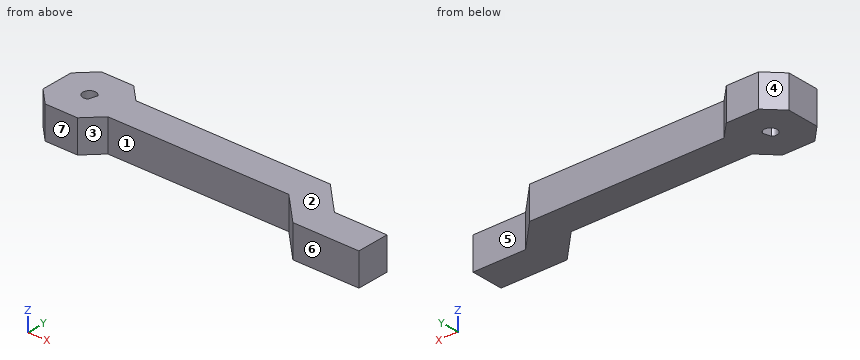
from build123d import *

# Parameters (mm, degrees)
BOSS_EXTRUDE1_DEPTH = 20


with BuildPart() as part:
    # Sketch1 → Boss-Extrude1 (new body)
    with BuildSketch(Plane.XY):
        Polygon((-125.92552771, 40.003004944), (-115.92552771, 50.003004944), (-95.92552771, 50.003004944), (-85.92552771, 40.003003647), (34.07447229, 40.003003647), (52.904699458, 21.17277648), (85.359896376, 21.17277648), (85.359896376, 1.17277648), (44.62042821, 1.17277648), (25.790201043, 20.003003647), (-85.92552771, 20.003003647), (-95.92552771, 10.003004944), (-115.92552771, 10.003004944), (-125.92552771, 20.003004944), align=None)
        with BuildLine():
            Line((-103.718736643, 26.666828512), (-102.339668887, 31.775465524))
            ThreePointArc((-102.339668887, 31.775465524), (-109.787294302, 31.04548218), (-103.718736643, 26.666828512))
        make_face(mode=Mode.SUBTRACT)
    extrude(amount=BOSS_EXTRUDE1_DEPTH)


solid = part.part
Could you check a few things on this model? Use its own coordinates, in mm. Face numbers are marked on the shaded views. A direction names the side the tool comes from. Give positions to 0.01 mm unless a question says otherwise; leave off trailing zeros. Order: outer loops, then holes, each group sorted by start corner. A loop starts at its lowest first (then second) coordinate and runs counter-clockwise, first axis right, second up. Notation, with made-up numbers: (74, 85) -> (101, 85) arc R16 cw to (101, 92) -> close; hole circle Ø6 at (-20, 74). An arc over 180 degrees is marked (long way). Answer in a Markdown table with one row per item. Add a question column.
Item 1: Imagine slicing it at B-B (z = 4.25). List the corners of the cut face in (x, y) for me.
Item 2: For the marked faces 5, 6 and 7, which set-ups out of +Z, -Z, +X, -X, +Y, -Y let a thin tool reach every point of the face, with its end or its side?
Item 3: I'm going to push flat-ended pins straight in: P1, Ø6, axis at x = -4.5, z = 8.5, coming from the +Y side; P2, Ø6, axis at x = 69, z = 10, coming from the +Y side; P3, Ø1, axis at y = 44, z = 12, coming from the +X side; P4, Ø5, axis at x = -105.93, y = 30, coming from the -Z side. Where does each tip first touch, or does it pass through?
Item 4: We'd pull the mould along X, two halves only. Please class the marked faces 1, 2, 3 and 4: pulls with the +X half, pulls with the -X half, needs draft (parallel to the pull), parting line crosses it, or undercut.
Item 5: Imagine slicing it at D-D (y = 6). List the corners of the cut face in (x, z) for me.
Item 6: Imagine slicing it at A-A (y = 16). List the corners of the cut face in (x, z) for me.
Item 7: Imagine slicing it at C-C (x = -100). List the corners of the cut face in (y, z) for me, and give its area (3 significant figures).
Item 8: Please list where these lines run through material, in increasing order: probe 1 along Y at (x, z) = (71, 15.75); probe 2 along Y at (x, z) = (22.5, 17.5); probe 3 along X at (y, z) = (13, 15.5).
Result:
| question | item | result |
|---|---|---|
| 1 | outline | (-125.93, 20) -> (-115.93, 10) -> (-95.93, 10) -> (-85.93, 20) -> (25.79, 20) -> (44.62, 1.17) -> (85.36, 1.17) -> (85.36, 21.17) -> (52.9, 21.17) -> (34.07, 40) -> (-85.93, 40) -> (-95.93, 50) -> (-115.93, 50) -> (-125.93, 40) -> close; hole (-103.72, 26.67) -> (-102.34, 31.78) arc R4 ccw (long way) to start |
| 2 | face 5 | +Z, -Z, +X, +Y |
| 2 | face 6 | +Z, -Z, +X, -X, -Y |
| 2 | face 7 | +Z, -Z, -X, -Y |
| 3 | P1 | y = 40 |
| 3 | P2 | y = 21.17 |
| 3 | P3 | x = -89.42 |
| 3 | P4 | through |
| 4 | face 1 | undercut |
| 4 | face 2 | needs draft |
| 4 | face 3 | undercut |
| 4 | face 4 | pulls with the -X half |
| 5 | outline | (39.79, 0) -> (85.36, 0) -> (85.36, 20) -> (39.79, 20) -> close |
| 6 | outline | (-121.92, 0) -> (-89.93, 0) -> (-89.93, 20) -> (-121.92, 20) -> close; (29.79, 0) -> (85.36, 0) -> (85.36, 20) -> (29.79, 20) -> close |
| 7 | outline | (10, 0) -> (50, 0) -> (50, 20) -> (10, 20) -> close |
| 7 | area | 800 mm2 |
| 8 | probe 1 | 1.17 to 21.17 |
| 8 | probe 2 | 20 to 40 |
| 8 | probe 3 | -118.92 to -92.93, 32.79 to 85.36 |
